The model under review builds one solid part; all positions refer to its coordinate system, in mm. Face numbers are marked on the shaded views. A direction names the side the tool comes from. Round coordinates to 2 decimals unless told otherwise and drop trailing zeros. Write each loop counter-clockwise with the first axis right and the second up, starting at its lowest first coordinate (ties: lowest second). Pieces come first, ordered by that corner, then holes. Notation, with made-up numbers: M 20,-29.5 L 69,-29.5 A17 ccw 69,-0.5 Z; hole C 20,20 d2. An arc over 180 degrees is marked long. One line per item, written item: value. Start each with the question number.
1) Mouldability with a two-part tool opening along X and no side actions: class the marked faces 1, 2 and 3 as +X half, -X half, draft (parallel to the pull), parting line (faces both ways), or undercut.
2) Take a section at A-A, the plane z = 255. Write out the cut boundary in (x, y).
3) For P1, Ø23, axis at x = 84, y = -48, coming from the +Z side, flat-tipped, find the tip position at first contact; note if it passes through.
4) Take a section at B-B, the plane z = 4.5. Write out the cut boundary in (x, y), and give its area (3 significant figures).
5) Tool access review of the marked faces 4 and 5: name each direction out of +Z, -Z, +X, -X, +Y, -Y from which nothing blocks a thin tool from reaching the whole face with its end or side.
6) Wall thickness on probe 1 along X at (y, z) = (-58.5, 112); probe 2 along X at (y, z) = (-6, 218.5); probe 3 along Y at (x, z) = (141, 90.5): over which ranges is each line inside the solid? List them lowest first.
7) Take a section at D-D, the plane y = -58. Write out the cut boundary in (x, z).
8) Take a section at C-C, the plane x = 192. Write out the cut boundary in (y, z), and give its area (3 significant figures).
from build123d import *

# Parameters (mm, degrees)
F0_W     = 330.2
F0_H     = 304.8
F1_DEPTH = 88.9
F2_W     = 317.5
F2_H     = 76.2
F3_DEPTH = 298.45
F5_DEPTH = 127


with BuildPart() as f1:
    # F0 (on Front) → F1 (new body)
    with BuildSketch(Plane.XZ):
        with Locations((58.008134, 136.263882)):
            Rectangle(F0_W, F0_H)
    extrude(amount=F1_DEPTH)

    # F2 (on face) → F3 (cut)
    with BuildSketch(Plane.XY.offset(288.663882)):
        with Locations((58.008134, -44.45)):
            Rectangle(F2_W, F2_H)
    extrude(amount=-F3_DEPTH, mode=Mode.SUBTRACT)

    # F4 (on face) → F5 (cut)
    with BuildSketch(Plane.XZ.offset(88.9)):
        with BuildLine():
            Line((-18.191866, 288.663882), (-18.191866, 136.263882))
            ThreePointArc((-18.191866, 136.263882), (58.008134, 60.063882), (134.208134, 136.263882))
            Line((134.208134, 136.263882), (134.208134, 288.663882))
            Line((134.208134, 288.663882), (-18.191866, 288.663882))
        make_face()
    extrude(amount=-F5_DEPTH, mode=Mode.SUBTRACT)


solid = f1.part
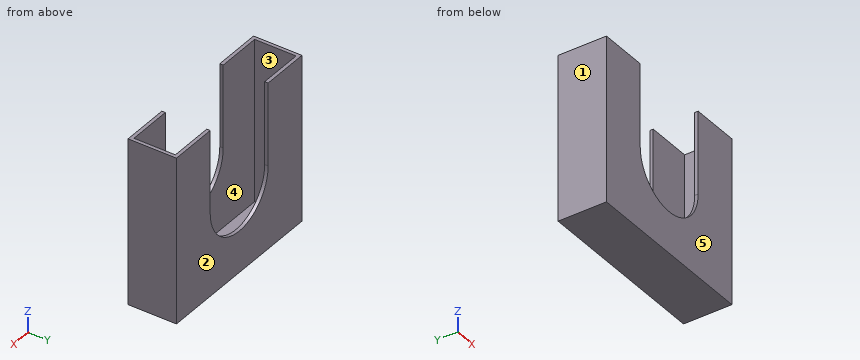
Checked values:
1. face 1: -X half
1. face 2: draft
1. face 3: undercut
2. outline: M -107.09,-88.9 L -18.19,-88.9 L -18.19,-82.55 L -100.74,-82.55 L -100.74,-6.35 L -18.19,-6.35 L -18.19,0 L -107.09,0 Z; M 134.21,-88.9 L 223.11,-88.9 L 223.11,0 L 134.21,0 L 134.21,-6.35 L 216.76,-6.35 L 216.76,-82.55 L 134.21,-82.55 Z
3. P1: stops at z = -9.79
4. outline: M -107.09,-88.9 L 223.11,-88.9 L 223.11,0 L -107.09,0 Z; hole M -100.74,-82.55 L 216.76,-82.55 L 216.76,-6.35 L -100.74,-6.35 Z
4. area: 5,160 mm2
5. face 4: +Z
5. face 5: +Z, -Z, +X, -X, -Y
6. probe 1: x = -107.09 to -100.74, 216.76 to 223.11
6. probe 2: x = -107.09 to -18.19, 134.21 to 223.11
6. probe 3: y = -88.9 to -82.55, -6.35 to 0
7. outline: M -107.09,-16.14 L 223.11,-16.14 L 223.11,288.66 L 216.76,288.66 L 216.76,-9.79 L -100.74,-9.79 L -100.74,288.66 L -107.09,288.66 Z
8. outline: M -88.9,-16.14 L 0,-16.14 L 0,288.66 L -6.35,288.66 L -6.35,-9.79 L -82.55,-9.79 L -82.55,288.66 L -88.9,288.66 Z
8. area: 4,350 mm2
